For this review, take the finished solid that the model builds, in its own axes (mm). A direction names the side the tool comes from. Coordinates: 2 decimals unless noted, no trailing zeros. Order: outer loops, then holes, each group sorted by start corner. A loop starts at its lowest first (then second) coordinate and runs counter-clockwise, first axis right, second up. Notation, with made-up numbers: (39.5, 10) - (65.5, 10) arc R29 cw to (65.5, 45) - close; hole circle Ø1 at (24, -36). An arc over 180 degrees is marked (long way). One line per item, written item: value. Start each with the question number.
(1) For faces 4 (the cylindrical face through (-28.52, -58.4, 3.25)), 5 (the cylindrical face through (-0.509, -69.304, 4.686)), 6 (the cylindrical face through (27.98, -58.4, 3.25)), 7 (the flat face through (28.229, -28, -17)), 8 (the flat face through (-28.771, -28, 17)), list the 3-axis set-ups (+Z, -Z, +X, -X, +Y, -Y) from which the entire face can be reached by the end or side of a thin tool; tool diameter is ignored.
(2) Mouldability with a two-part tool opening along Z and no side actions: class faces 1 (the cylindrical face through (0.128, -16.526, 3.794)), 2 (the flat face through (-26.271, -7, -9)), 3 (the cylindrical face through (21.166, 6.415, 8.888)) as released by +Z, released by -Z, zero draft, split by the parting line, or undercut.
(3) Consider section B-B on z = -32. Write out the cut boundary in (x, y), then the cut area to 3 significant figures.
(4) To check wall thickness, follow line 1 along X through (y, z) = (0.5, 14.5); line 2 along Y through (x, z) = (0, 0); line 3 along X through (y, z) = (-60, -13.5). State the ranges of each line that lie inside material, in increasing order.
(5) Consider section A-A on z = 0. Write out the cut boundary in (x, y), then the cut area to 3 significant figures.
(6) Consider section C-C on x = -4. Write out the cut boundary in (y, z).
(7) Clearance check with flat-ended pins moving along their axes: pin 1 (6 mm diameter, centred on x = -14, y = -14.5, fed in from -Z); pin 2 (12 mm diameter, centred on x = 10, z = 28, fed in from -Y); pin 3 (6 mm diameter, centred on x = -1.5, z = 20, fed in from -Y). State where each tip first meets the part, or that it passes through.
(8) Consider section D-D on y = -3.5. Write out the cut boundary in (x, z).
```python
from build123d import *

# Parameters (mm, degrees)
FILLET1_R = 2


with BuildPart() as part:
    # Sketch1 → Revolve1 (revolve)
    with BuildSketch(Plane.XY, mode=Mode.PRIVATE) as revolve1_sk:
        Polygon((28.229021504, -16.110191686), (28.229021504, -8.610191686), (25.729021504, -8.610191686), (25.729021504, 7.389808314), (16.729021504, 7.389808314), (16.729021504, 2.389808314), (-17.270978496, 2.389808314), (-17.270978496, 7.389808314), (-26.270978496, 7.389808314), (-26.270978496, -8.610191686), (-28.770978496, -8.610191686), (-28.770978496, -16.110191686), align=None)
    revolve(revolve1_sk.sketch.rotate(Axis((27.520922354, -33.610191686, 0), (-1, 0, 0)), 90), axis=Axis((27.520922354, -33.610191686, 0), (-1, 0, 0)))

    # Fillet1
    fillet1_edges = [part.edges().sort_by_distance(p)[0] for p in [
        (-26.270978496, -33.610191686, 25),
        (25.729021504, -33.610191686, 25),
    ]]
    fillet(fillet1_edges, radius=FILLET1_R)


solid = part.part
```
Geometry check:
1. face 4: -X
1. face 5: none
1. face 6: +X
1. face 7: +Z, -Z, +X, +Y, -Y
1. face 8: +Z, -Z, -X, +Y, -Y
2. face 1: undercut
2. face 2: zero draft
2. face 3: split by the parting line
3. outline: (-26.27, -59.24) - (-17.27, -59.24) - (-17.27, -50.1) - (16.73, -50.1) - (16.73, -59.24) - (25.73, -59.24) - (25.73, -7.98) - (16.73, -7.98) - (16.73, -17.12) - (-17.27, -17.12) - (-17.27, -7.98) - (-26.27, -7.98) - close
3. area: 2,040 mm^2
4. line 1: x = -26.27 to -17.27, 16.73 to 25.73
4. line 2: y = -69.61 to -51.11, -16.11 to 2.39
4. line 3: x = -26.27 to 25.73
5. outline: (-28.77, -58.61) - (-28.27, -58.61) arc R2 cw to (-26.27, -60.61) - (-26.27, -74.61) - (-17.27, -74.61) - (-17.27, -69.61) - (16.73, -69.61) - (16.73, -74.61) - (25.73, -74.61) - (25.73, -60.61) arc R2 cw to (27.73, -58.61) - (28.23, -58.61) - (28.23, -51.11) - (-28.77, -51.11) - close; (-28.77, -16.11) - (28.23, -16.11) - (28.23, -8.61) - (27.73, -8.61) arc R2 cw to (25.73, -6.61) - (25.73, 7.39) - (16.73, 7.39) - (16.73, 2.39) - (-17.27, 2.39) - (-17.27, 7.39) - (-26.27, 7.39) - (-26.27, -6.61) arc R2 cw to (-28.27, -8.61) - (-28.77, -8.61) - close
5. area: 2,180 mm^2
6. outline: circle Ø72 at (-33.61, 0); hole circle Ø35 at (-33.61, 0)
7. pin 1: stops at z = -32.19
7. pin 2: stops at y = -62.11
7. pin 3: stops at y = -65.34
8. outline: (-26.27, -27.83) - (-17.27, -27.83) - (-17.27, -19.73) - (16.73, -19.73) - (16.73, -27.83) - (25.73, -27.83) - (25.73, 27.83) - (16.73, 27.83) - (16.73, 19.73) - (-17.27, 19.73) - (-17.27, 27.83) - (-26.27, 27.83) - close
